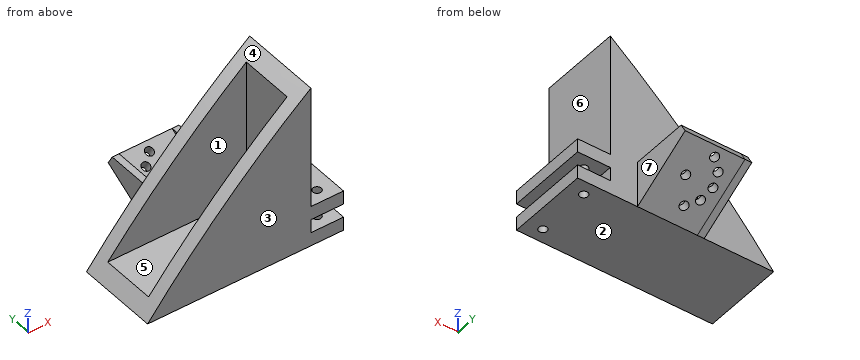
```python
from build123d import *

# Parameters (mm, degrees)
EXTRUDE_1_DEPTH          = 30
CUT_EXTRUDE_1_DEPTH      = 98.124713642
CUT_EXTRUDE_1_DEPTH_BACK = 98.124713642
SKETCH_2_R               = 1.55
CUT_EXTRUDE_6_DEPTH      = 10
EXTRUDE_3_DEPTH          = 12.5
SKETCH_12_W              = 5
SKETCH_12_H              = 30
EXTRUDE_4_DEPTH          = 2
SKETCH_14_W              = 22
SKETCH_14_H              = 27
SKETCH_14_R              = 1.55
EXTRUDE_5_DEPTH          = 4
EXTRUDE_8_DEPTH          = 2.5
EXTRUDE_9_DEPTH          = 2.5


with BuildPart() as part:
    # 草图1 → 凸台-拉伸1 (new body)
    with BuildSketch(Plane(origin=(0, 0, 0), x_dir=(1, 0, 0), z_dir=(0, 1, 0))):
        with BuildLine():
            Line((0, 0), (-70, 0))
            ThreePointArc((-70, 0), (-41.606545869, -31.737243891), (-10, -60.276114672))
            Line((-10, -60.276114672), (-10, -15))
            Line((-10, -15), (0, -15))
            Line((0, -15), (0, -10))
            Line((0, -10), (-10, -10))
            Line((-10, -10), (-10, -5))
            Line((-10, -5), (0, -5))
            Line((0, -5), (0, 0))
        make_face()
    extrude(amount=EXTRUDE_1_DEPTH)

    # 草图2 → 切除-拉伸1 (cut, two sides: drawn at the far end of the back side and taken through both)
    with BuildSketch(Plane(origin=(0, 0, 0), x_dir=(-1, 0, 0), z_dir=(0, 0, -1)).offset(-CUT_EXTRUDE_1_DEPTH_BACK)):
        with Locations((4, 25)):
            Circle(SKETCH_2_R)
        with Locations((4, 5)):
            Circle(SKETCH_2_R)
    extrude(amount=CUT_EXTRUDE_1_DEPTH + CUT_EXTRUDE_1_DEPTH_BACK, mode=Mode.SUBTRACT)

    # 草图9 → 切除-拉伸6 (cut, symmetric)
    with BuildSketch(Plane(origin=(0, 15, 0), x_dir=(1, 0, 0), z_dir=(0, 1, 0))):
        with BuildLine():
            Line((-65.918016471, -5), (-59.391772218, -5))
            Line((-59.391772218, -5), (-15, -5))
            Line((-15, -5), (-15, -15))
            Line((-15, -15), (-15, -49.60330608))
            Line((-15, -49.60330608), (-15, -56.155472209))
            ThreePointArc((-15, -56.155472209), (-41.615194331, -31.728555364), (-65.918016471, -5))
        make_face()
    extrude(amount=CUT_EXTRUDE_6_DEPTH, both=True, mode=Mode.SUBTRACT)

    # 草图11 → 凸台-拉伸3 (add, symmetric)
    with BuildSketch(Plane(origin=(0, 15, 0), x_dir=(1, 0, 0), z_dir=(0, 1, 0))):
        Polygon((-15, -5), (-23, -5), (-15, -10), align=None)
    extrude(amount=EXTRUDE_3_DEPTH, both=True)

    # 草图12 → 凸台-拉伸4 (add)
    with BuildSketch(Plane(origin=(0, 0, 0), x_dir=(0, 0, -1), z_dir=(1, 0, 0))):
        with Locations((-12.5, 15)):
            Rectangle(SKETCH_12_W, SKETCH_12_H)
        with Locations((-2.5, 15)):
            Rectangle(SKETCH_12_W, SKETCH_12_H)
    extrude(amount=EXTRUDE_4_DEPTH)

    # 草图14 → 凸台-拉伸5 (add)
    with BuildSketch(Plane(origin=(0, 7.5, -12.990381057), x_dir=(-1, 0, 0), z_dir=(0, 0.499999999999998, -0.8660254037844398))):
        with Locations((31, 39.480762114)):
            Rectangle(SKETCH_14_W, SKETCH_14_H)
        with Locations(Location((28, 40.980762114, 0), (0, 0, 90))):
            Circle(SKETCH_14_R, mode=Mode.SUBTRACT)
        with Locations(Location((33, 49.641016151, 0), (0, 0, 90))):
            Circle(SKETCH_14_R, mode=Mode.SUBTRACT)
        with Locations(Location((36.660254038, 45.980762114, 0), (0, 0, 90))):
            Circle(SKETCH_14_R, mode=Mode.SUBTRACT)
        with Locations(Location((38, 40.980762114, 0), (0, 0, 90))):
            Circle(SKETCH_14_R, mode=Mode.SUBTRACT)
        with Locations(Location((36.660254038, 35.980762114, 0), (0, 0, 90))):
            Circle(SKETCH_14_R, mode=Mode.SUBTRACT)
        with Locations(Location((33, 32.320508076, 0), (0, 0, 90))):
            Circle(SKETCH_14_R, mode=Mode.SUBTRACT)
    extrude(amount=-EXTRUDE_5_DEPTH)

    # 草图18 → 凸台-拉伸8 (add)
    with BuildSketch(Plane(origin=(-20, 0, 0), x_dir=(0, 0, -1), z_dir=(1, 0, 0))):
        Polygon((-16.964101615, 51.382685902), (-4.618802154, 30), (-16.964101615, 30), align=None)
    extrude(amount=-EXTRUDE_8_DEPTH)

    # 草图19 → 凸台-拉伸9 (add)
    with BuildSketch(Plane.ZY.offset(42)):
        Polygon((0, 30), (13.5, 53.382685902), (16.964101615, 51.382685902), (16.964101615, 30), align=None)
    extrude(amount=EXTRUDE_9_DEPTH)


solid = part.part
```
Part model, mm, in its own coordinate system. Face numbers are marked on the shaded views. A direction names the side the tool comes from. Round coordinates to 2 decimals unless told otherwise and drop trailing zeros. Loops run counter-clockwise (first coordinate to the right, second up) from the corner with the lowest first, then second, coordinate; pieces in that order, holes last.
1. Slice it at D-D (x = -52). Give the cut face in (y, z).
Solutions:
outline: (0, 0) - (30, 0) - (30, 20.9) - (25, 20.9) - (25, 5) - (5, 5) - (5, 20.9) - (0, 20.9) - close
2. 3-axis set-ups, long thin cutter, end or side, ignore diameter. For the marked faces 4, 5, 6 and 7: which of +Z, -Z, +X, -X, +Y, -Y reach the whole face in a straight line?
Solutions:
face 4: +Z, -X, +Y, -Y
face 5: +Z, -X
face 6: +Z, +X, +Y, -Y
face 7: +Z, -Z, +X, +Y
3. Two-plate mould, pull along Y, no slides. Class the marked faces 1, 2 and 3: pulls with the +Y half, pulls with the -Y half, needs draft (parallel to the pull), parting line crosses it, or undercut.
Solutions:
face 1: undercut
face 2: needs draft
face 3: pulls with the -Y half
4. Drill centre lines: line 1 along Y through (x, z) = (-4, 1.25); line 2 along Y through (x, z) = (-30, 14); line 3 along Z through (x, y) = (-3, 27). Where is each one in solid material? Low to high.
Solutions:
line 1: y = 0 to 3.45, 6.55 to 23.45, 26.55 to 30
line 2: y = 0 to 5, 25 to 30, 46.25 to 53.09
line 3: z = 0 to 5, 10 to 15
5. Slice it at A-A (x = -7). Give the cut face in (y, z).
Solutions:
outline: (0, 0) - (30, 0) - (30, 5) - (0, 5) - close; (0, 10) - (30, 10) - (30, 15) - (0, 15) - close
6. Slice it at C-C (z = 38). Give the cut face in (x, y).
Solutions:
outline: (-35.23, 0) - (-10, 0) - (-10, 30) - (-35.23, 30) - (-35.23, 25) - (-15, 25) - (-15, 5) - (-35.23, 5) - close
7. Slice it at B-B (y = 27.5). Give the cut face in (x, z), and give its area (3 significant figures).
Solutions:
outline: (-70, 0) - (2, 0) - (2, 5) - (-10, 5) - (-10, 10) - (2, 10) - (2, 15) - (-10, 15) - (-10, 60.28) arc R400 ccw to start
area: 2,060 mm2
8. Flat gauge pins, fed straight in: pin 1 (10 mm diameter, centred on y = 13.5, z = 8, fed in from -X); pin 2 (0.8 mm diameter, centred on x = -21.5, y = 39, fed in from +Z); pin 3 (3.5 mm diameter, centred on x = -4, y = 5, fed in from +Z). Where does each tip first touch, or does it go through?
Solutions:
pin 1: stops at x = -67.57
pin 2: stops at z = 16.96
pin 3: stops at z = 15
